from build123d import *

# Parameters (mm, degrees)
SKETCH1_W           = 75
SKETCH1_H           = 52.75
BOSS_EXTRUDE1_DEPTH = 1.1
SKETCH2_R           = 1.185
CUT_EXTRUDE1_DEPTH  = 46.859575063
SKETCH3_W           = 74.6
SKETCH3_H           = 45
BOSS_EXTRUDE2_DEPTH = 6
SKETCH4_W           = 60.4
SKETCH4_H           = 32.75
CUT_EXTRUDE2_DEPTH  = 0.5


with BuildPart() as part:
    # Sketch1 → Boss-Extrude1 (new body)
    with BuildSketch(Plane.XY):
        Rectangle(SKETCH1_W, SKETCH1_H)
    extrude(amount=BOSS_EXTRUDE1_DEPTH)

    # Sketch2 → Cut-Extrude1 (cut, through all)
    with BuildSketch(Plane.XY.offset(1.1)):
        with Locations((-35, -24.125)):
            Circle(SKETCH2_R)
        with Locations((35, -24.125)):
            Circle(SKETCH2_R)
        with Locations((35, 26.375)):
            Circle(SKETCH2_R)
        with Locations((-35, 26.375)):
            Circle(SKETCH2_R)
    extrude(amount=-CUT_EXTRUDE1_DEPTH, mode=Mode.SUBTRACT)

    # Sketch3 → Boss-Extrude2 (add)
    with BuildSketch(Plane.XY.offset(1.1)):
        with Locations((0, 1.095)):
            Rectangle(SKETCH3_W, SKETCH3_H)
    extrude(amount=BOSS_EXTRUDE2_DEPTH)

    # Sketch4 → Cut-Extrude2 (cut)
    with BuildSketch(Plane.XY.offset(7.1)):
        with Locations((0, 1.22)):
            Rectangle(SKETCH4_W, SKETCH4_H)
    extrude(amount=-CUT_EXTRUDE2_DEPTH, mode=Mode.SUBTRACT)


solid = part.part
CAD build for the part. Positions are in the model's coordinates, mm. A direction names the side the tool comes from. Give positions to 0.01 mm unless a question says otherwise; leave off trailing zeros. Loops run counter-clockwise (first coordinate to the right, second up) from the corner with the lowest first, then second, coordinate; pieces in that order, holes last. Notation, with made-up numbers: M -10.75,80.5 L 13.25,80.5 A9 cw 13.25,86.5 Z; hole C -38,-34.5 d5. An arc over 180 degrees is marked long. Answer in a Markdown table with one row per item. Add a question column.
Item 1: Drop flat-ended pins along their axis: P1, Ø0.6, axis at x = -2.5, z = 7, coming from the +Y side (3 decimals); P2, Ø5, axis at x = 7.5, y = 7.5, coming from the +Z side; P3, Ø2.5, axis at x = -35, y = -24.125, coming from the +Z side. Give the stop position or say it passes through.
Item 2: Band-saw the part on A-A on x = 35. Give the cut face in (y, z) (3 decimals).
Item 3: Band-saw the part on B-B on y = -6.5. Give the cut face in (x, z).
Item 4: Probe probe 1 along Y at (x, z) = (-35, 0.65) (3 decimals); probe 2 along Z at (x, y) = (23, -2); probe 3 along Y at (x, z) = (2.5, 2.5) (3 decimals). List the from-to ranges inside material, lowest first.
Item 5: Tool access for faces 1 (the face through (35.5, -25.2, 0.6)), 2 (the face through (0, 1, 6.6)), 3 (the face through (-1, -19, 7.1)), 4 (the face through (-1, -21.405, 4)), 5 (the face through (-1, 23.595, 4)): list every direction of +Z, -Z, +X, -X, +Y, -Y with a clear straight run to the whole face (end or side of a thin tool).
Item 6: Band-saw the part on C-C on z = 3. Give the cut face in (x, y) (3 decimals), then the cut area to 3 significant figures.
Item 7: Band-saw the part on D-D on x = 16. Give the cut face in (y, z) (3 decimals), then the cut area to 3 significant figures.
Item 8: Mould opens along X. For faces 6 (the face through (-37.3, 1, 4)), 7 (the face through (-1, 0, 0)), 8 (the face through (-34.5, -25.2, 0.6)), 9 (the face through (37.3, 1, 4)) say: +X half, -X half, draft (parallel to the pull), parting line (faces both ways), or undercut.
Reply:
| question | item | result |
|---|---|---|
| 1 | P1 | stops at y = 23.595 |
| 1 | P2 | stops at z = 6.6 |
| 1 | P3 | stops at z = 1.1 |
| 2 | outline | M -26.375,0 L -25.31,0 L -25.31,1.1 L -26.375,1.1 Z; M -22.94,0 L 25.19,0 L 25.19,1.1 L 23.595,1.1 L 23.595,7.1 L -21.405,7.1 L -21.405,1.1 L -22.94,1.1 Z |
| 3 | outline | M -37.5,0 L 37.5,0 L 37.5,1.1 L 37.3,1.1 L 37.3,7.1 L 30.2,7.1 L 30.2,6.6 L -30.2,6.6 L -30.2,7.1 L -37.3,7.1 L -37.3,1.1 L -37.5,1.1 Z |
| 4 | probe 1 | y = -26.375 to -25.31, -22.94 to 25.19 |
| 4 | probe 2 | z = 0 to 6.6 |
| 4 | probe 3 | y = -21.405 to 23.595 |
| 5 | face 1 | +Z, -Z |
| 5 | face 2 | +Z |
| 5 | face 3 | +Z, +X, -X, +Y, -Y |
| 5 | face 4 | +Z, +X, -X, -Y |
| 5 | face 5 | +Z, +X, -X, +Y |
| 6 | outline | M -37.3,-21.405 L 37.3,-21.405 L 37.3,23.595 L -37.3,23.595 Z |
| 6 | area | 3,360 mm^2 |
| 7 | outline | M -26.375,0 L 26.375,0 L 26.375,1.1 L 23.595,1.1 L 23.595,7.1 L 17.595,7.1 L 17.595,6.6 L -15.155,6.6 L -15.155,7.1 L -21.405,7.1 L -21.405,1.1 L -26.375,1.1 Z |
| 7 | area | 312 mm^2 |
| 8 | face 6 | -X half |
| 8 | face 7 | draft |
| 8 | face 8 | undercut |
| 8 | face 9 | +X half |
